Can you work these out from the model? Positions are in its coordinate system, mm. Face numbers are marked on the shaded views. A direction names the side the tool comes from. Coordinates: 2 decimals unless noted, no trailing zeros. Write each loop counter-clockwise with the first axis right and the second up, starting at its lowest first coordinate (ties: lowest second). Pieces come first, ordered by that corner, then holes. Notation, with made-up numbers: (69, 8.25) -> (113, 8.25) arc R7 ccw to (113, 20.25) -> close; hole circle Ø10 at (62.25, 14.5). An arc over 180 degrees is marked (long way). Use one line per item in the form item = value.
```python
from build123d import *

# Parameters (mm, degrees)
PAD_DEPTH       = 8.65
SKETCH001_R     = 1.625
PAD001_DEPTH    = 3.7
PAD002_DEPTH    = 3
POCKET_START    = -2
POCKET_DEPTH    = 8.3
POCKET001_DEPTH = 73.3327090398


with BuildPart() as part:
    # Sketch → Pad (new body, symmetric)
    with BuildSketch(Plane.XZ):
        with BuildLine():
            ThreePointArc((0, -3.15), (3.1491038588, 0.075132459), (-0.1502221693, 3.1464159451))
            Line((-16.9622926765, 2.3437421264), (-0.1502221693, 3.1464159451))
            ThreePointArc((-16.9622926765, 2.3437421264), (-20.6807417475, 0.6452200383), (-22.2, -3.15))
            Line((0, -3.15), (-22.2, -3.15))
        make_face()
    extrude(amount=PAD_DEPTH, both=True)

    # Sketch001 (on Face6 of Pad) → Pad001 (join)
    with BuildSketch(Plane.XZ.offset(8.65)):
        Circle(SKETCH001_R)
    pad001 = extrude(amount=PAD001_DEPTH)

    # Sketch002 → Pad002 (join)
    with BuildSketch(Plane.YZ):
        with BuildLine():
            ThreePointArc((-8.65, 1), (-9.65, 0), (-8.65, -1))
            Line((-8.65, -1), (-8.65, 1))
        make_face()
    pad002 = extrude(amount=PAD002_DEPTH)

    # Sketch003 (on Face5 of Pad002) → Pocket (cut)
    with BuildSketch(Plane.XZ.offset(8.65).offset(POCKET_START)):
        with BuildLine():
            Line((-21.7833060109, -1.05), (0, -1.05))
            ThreePointArc((0, -1.05), (1.8482397845, 0.4106515201), (0.8542561404, 2.5464159451))
            Line((1.8542561404, 2.5464159451), (0.8542561404, 2.5464159451))
            ThreePointArc((1.8542561404, 2.5464159451), (0.9032900662, 3.0177089085), (-0.1502221693, 3.1464159451))
            Line((-16.9622926765, 2.3437421264), (-0.1502221693, 3.1464159451))
            ThreePointArc((-16.9622926765, 2.3437421264), (-19.8659481576, 1.3474183998), (-21.7833060109, -1.05))
        make_face()
    pocket = extrude(amount=-POCKET_DEPTH, mode=Mode.SUBTRACT)

    # Sketch004 (on Face12 of Pocket) → Pocket001 (cut, through all)
    with BuildSketch(Plane(origin=(0, 0, -3.15), x_dir=(1, 0, 0), z_dir=(0, 0, -1))):
        with BuildLine():
            ThreePointArc((-10, 6.65), (-11.2, 5.45), (-10, 4.25))
            Line((-10, 4.25), (5, 4.25))
            Line((5, 4.25), (5, 6.65))
            Line((5, 6.65), (-10, 6.65))
        make_face()
    pocket001 = extrude(amount=-POCKET001_DEPTH, mode=Mode.SUBTRACT)

    # Mirrored: Pocket001, Pocket, Pad002, Pad001 across XZ
    add(pocket001.mirror(Plane.XZ), mode=Mode.SUBTRACT)
    add(pocket.mirror(Plane.XZ), mode=Mode.SUBTRACT)
    add(pad002.mirror(Plane.XZ))
    add(pad001.mirror(Plane.XZ))


solid = part.part
```
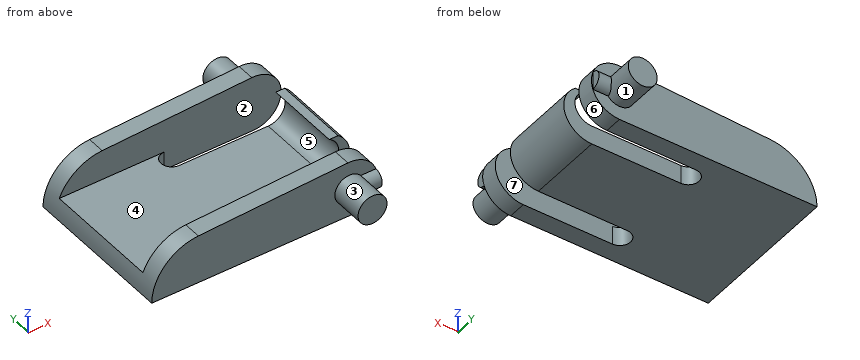
Q1. Suppose I cut it at D-D (z = -2.25). Write out the boundary of the cut face in (x, y).
Return value:
outline = (-22.13, -8.65) -> (2.2, -8.65) -> (2.2, -6.65) -> (-10, -6.65) arc R1.2 cw to (-10, -4.25) -> (2.2, -4.25) -> (2.2, 4.25) -> (-10, 4.25) arc R1.2 cw to (-10, 6.65) -> (2.2, 6.65) -> (2.2, 8.65) -> (-22.13, 8.65) -> close
Q2. Will these pins go through, and if not, where does the flat tip stop? pin 1 (5 mm diameter, centred on x = 0.5, y = 0, fed in from +Z); pin 2 (3 mm diameter, centred on x = -4.5, y = 5.5, fed in from +Z); pin 3 (1 mm diameter, centred on x = -13.5, z = 1, fed in from -Y).
Return value:
pin_1 = 2.55
pin_2 = 2.98
pin_3 = -8.65
Q3. Suppose I cut it at B-B (x = -16). Write out the boundary of the cut face in (y, z).
Return value:
outline = (-8.65, -3.15) -> (8.65, -3.15) -> (8.65, 2.39) -> (6.65, 2.39) -> (6.65, -1.05) -> (-6.65, -1.05) -> (-6.65, 2.39) -> (-8.65, 2.39) -> close
Q4. For the marked faces 1, 2, 3 and 4, which set-ups out of +Z, -Z, +X, -X, +Y, -Y let a thin tool reach every point of the face, with its end or its side?
Return value:
face_1 = +Y
face_2 = +Z, +X
face_3 = -Y
face_4 = +Z, -X
Q5. Suppose I cut it at C-C (y = 10.5). Write out the boundary of the cut face in (x, z) (3 decimals), then the cut area to 3 significant figures.
Return value:
outline = circle Ø3.25 at (0, 0)
area = 8.30 mm2
Q6. Suppose I cut it at A-A (z = 0). Write out the boundary of the cut face in (x, y) (3 decimals), then the cut area to 3 significant figures.
Return value:
outline = (-21.209, -8.65) -> (-1.625, -8.65) -> (-1.625, -12.35) -> (1.625, -12.35) -> (1.625, -9.65) -> (3, -9.65) -> (3, -8.65) -> (3.15, -8.65) -> (3.15, -6.65) -> (-21.209, -6.65) -> close; (-21.209, 6.65) -> (3.15, 6.65) -> (3.15, 8.65) -> (3, 8.65) -> (3, 9.65) -> (1.625, 9.65) -> (1.625, 12.35) -> (-1.625, 12.35) -> (-1.625, 8.65) -> (-21.209, 8.65) -> close; (1.699, -4.25) -> (3.15, -4.25) -> (3.15, 4.25) -> (1.699, 4.25) -> close
area = 137 mm2
Q7. Thinking about a two-plate mould opening in Z: for the marked faces 5, 6 and 7, which applies, released by +Z, released by -Z, zero draft, split by the parting line, or undercut?
Return value:
face_5 = undercut
face_6 = split by the parting line
face_7 = zero draft
Q8. If I drill on line 1 (Y direction, x = -6.75, z = 0.25); line 2 (Y direction, x = 1.75, z = 0); line 3 (Z direction, x = -13.5, y = 5), over which ranges is the centre line in solid material (lowest first)? Write a range as from..to.
Return value:
line_1 = -8.65..-6.65, 6.65..8.65
line_2 = -9.65..-6.65, -4.25..4.25, 6.65..9.65
line_3 = -3.15..-1.05
